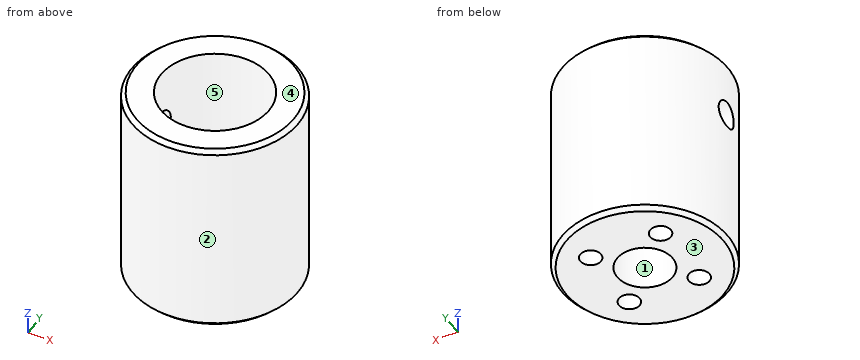
```python
from build123d import *

# Parameters (mm, degrees)
SKETCH_1_R                  = 10
EXTRUDE_1_DEPTH             = 24
SKETCH_2_R                  = 6.5
CUT_EXTRUDE_1_DEPTH         = 15
M4X0_71_D                   = 3.3
M4X0_71_DEPTH               = 5
M4X0_71_TIP                 = 0.991420021
M3X0_51_OUTLINE_R           = 1.25
M3X0_51_DEPTH               = 9
HOLE_WIZARD_M31_D           = 3.4
HOLE_WIZARD_M31_CBORE_D     = 6.7
HOLE_WIZARD_M31_CBORE_DEPTH = 6
CHAMFER_1_SIZE              = 0.5


# Read off the part's stored shape, not the designer's step: Отверстие обработанное метчиком M3x0.51
with BuildPart() as part:
    # Эскиз1 → Бобышка-Вытянуть1 (new body)
    with BuildSketch(Plane.XY):
        Circle(SKETCH_1_R)
    extrude(amount=EXTRUDE_1_DEPTH)

    # Эскиз2 → Вырез-Вытянуть1 (cut)
    with BuildSketch(Plane.XY.offset(24)):
        Circle(SKETCH_2_R)
    extrude(amount=-CUT_EXTRUDE_1_DEPTH, mode=Mode.SUBTRACT)

    # Отверстие обработанное метчиком M4x0.71
    with Locations(Plane(origin=(-10, 0, 0), x_dir=(0, 0, -1), z_dir=(-1, 0, 0))):
        with Locations((-17, 0)):
            Hole(M4X0_71_D / 2, depth=M4X0_71_DEPTH)
            with Locations((0, 0, -(M4X0_71_DEPTH + M4X0_71_TIP / 2))):  # 118° drill point
                Cone(0, M4X0_71_D / 2, M4X0_71_TIP, mode=Mode.SUBTRACT)

    # Отверстие обработанное метчиком M3x0.51 outline → Отверстие обработанное метчиком M3x0.51 (cut)
    with BuildSketch(Plane.XY):
        with Locations((4.242640687, -4.242640687)):
            Circle(M3X0_51_OUTLINE_R)
        with Locations((-4.242640687, -4.242640687)):
            Circle(M3X0_51_OUTLINE_R)
        with Locations((-4.242640687, 4.242640687)):
            Circle(M3X0_51_OUTLINE_R)
        with Locations((4.242640687, 4.242640687)):
            Circle(M3X0_51_OUTLINE_R)
    extrude(amount=M3X0_51_DEPTH, mode=Mode.SUBTRACT)

    # Цековка для  винта с полукруглой головкой M31 (through all)
    with Locations(Plane(origin=(0, 0, 0), x_dir=(-1, 0, 0), z_dir=(0, 0, -1))):
        with Locations((0, 0)):
            CounterBoreHole(HOLE_WIZARD_M31_D / 2, HOLE_WIZARD_M31_CBORE_D / 2, HOLE_WIZARD_M31_CBORE_DEPTH)

    # Фаска1
    chamfer_1_edges = [part.edges().sort_by_distance(p)[0] for p in [
        (-10, 0, 0),
        (-10, 0, 24),
    ]]
    chamfer(chamfer_1_edges, length=CHAMFER_1_SIZE)


solid = part.part
```
Can you work these out from the model? Positions are in its coordinate system, mm. Face numbers are marked on the shaded views. A direction names the side the tool comes from. Round coordinates to 2 decimals unless told otherwise and drop trailing zeros. Loops run counter-clockwise (first coordinate to the right, second up) from the corner with the lowest first, then second, coordinate; pieces in that order, holes last. Notation, with made-up numbers: M 83,37 L 126,37 A25 ccw 126,53 Z; hole C 2,49.25 d1. An arc over 180 degrees is marked long. Write item = value, one per line. Start each with the question number.
(1) Which directions (+Z, -Z, +X, -X, +Y, -Y) give clear straight access to the entire face, cutting with the end or side of a thin tool? Please do the marked faces 4 and 5.
(2) Suppose I cut it at A-A on x = 0. Write out the boundary of the cut face in (y, z).
(3) I need wall thicknesses on line 1 along Y through (x, z) = (4.5, 2); line 2 along Y through (x, z) = (0, 2); line 3 along Y through (x, z) = (0.25, 11.75). Which ranges of each line are inside material? Lowest first, please.
(4) I'm going to push flat-ended pins straight in: P1, Ø2, axis at x = 4.24, y = -4.24, coming from the -Z side; P2, Ø4, axis at y = 0, z = 17, coming from the -X side; P3, Ø1, axis at x = 2.5, z = 9.5, coming from the -Y side; P4, Ø6, axis at y = -6, z = 19.5, coming from the +X side. Where does each tip first touch, or does it pass through?
(5) If we mould it in two halves opening along Y, with no side actions, what happens to the marked faces 1, 2 and 3? For each: released by +Y, released by -Y, zero draft, split by the parting line, or undercut.
(6) Suppose I cut it at D-D on y = 1. Give the number of separate pieces and of enclosed holes in the cut face, plus the area to 3 significant figures.
(7) Suppose I cut it at C-C on z = 10. Write out the boundary of the cut face in (x, y), plus the area to 3 significant figures.
(8) Suppose I cut it at B-B on z = 4. Write out the boundary of the cut face in (x, y), plus the area to 3 significant figures.
Answer block:
q1.face_4 = +Z, +X, -X, +Y, -Y
q1.face_5 = +Z
q2.outline = M -10,0.5 L -9.5,0 L -3.35,0 L -3.35,6 L -1.7,6 L -1.7,9 L -6.5,9 L -6.5,24 L -9.5,24 L -10,23.5 Z; M 1.7,6 L 3.35,6 L 3.35,0 L 9.5,0 L 10,0.5 L 10,23.5 L 9.5,24 L 6.5,24 L 6.5,9 L 1.7,9 Z
q3.line_1 = -8.93 to -5.47, -3.02 to 3.02, 5.47 to 8.93
q3.line_2 = -10 to -3.35, 3.35 to 10
q3.line_3 = -10 to -6.5, 6.5 to 10
q4.P1 = 9
q4.P2 = -10
q4.P3 = -9.8
q4.P4 = 9.54
q5.face_1 = undercut
q5.face_2 = split by the parting line
q5.face_3 = zero draft
q6.separate_pieces = 3
q6.enclosed_holes = 0
q6.area = 229 mm²
q7.outline = C 0,0 d20; hole C 0,0 d13
q7.area = 181 mm²
q8.outline = C 0,0 d20; hole C -4.24,-4.24 d2.5; hole C -4.24,4.24 d2.5; hole C 0,0 d6.7; hole C 4.24,-4.24 d2.5; hole C 4.24,4.24 d2.5
q8.area = 259 mm²
